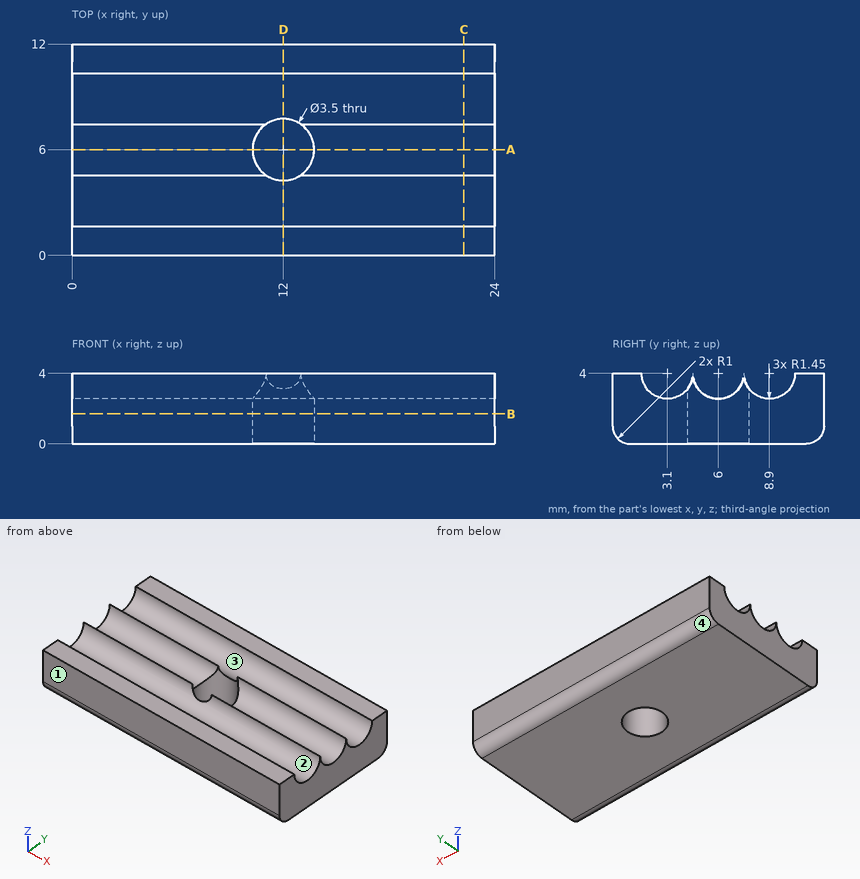
Design review of the part shown in the three views and the two pictorial views. Dimensions are in mm from the part's minimum x, y and z. Round coordinates to 2 decimals unless told otherwise and drop trailing zeros. Write each loop counter-clockwise with the first axis right and the second up, starting at its lowest first coordinate (ties: lowest second). Pieces come first, ordered by that corner, then holes. Notation, with made-up numbers: (53, 2.5) -> (59, 2.5) arc R21 cw to (59, 39.5) -> close; hole circle Ø7 at (87.5, -35.5). An arc over 180 degrees is marked (long way). Use one line per item in the form item = value.
1) Clearance check with a flat-ended pin moving along its axis: pin 1 (2 mm diameter, centred on x = 6, y = 6, fed in from +Z). State where the tip first meets the part, or that it passes through.
Found:
pin_1 = 2.95
2) To check wall thickness, follow L1, parallel to X at y = 6, z = 1.5; L2, parallel to Y at x = 12, z = 2.3; L3, parallel to Y at x = 10.75, z = 2.7. State the ranges of each line that lie inside material, in increasing order. Write a range as from..to.
Found:
L1 = 0..10.25, 13.75..24
L2 = 0..4.25, 7.75..12
L3 = 0..2.46, 3.74..4.78, 7.22..8.26, 9.54..12
3) Take a section at C-C, the plane x = 22.25. Write out the cut boundary in (y, z), and give its area (3 significant figures).
Found:
outline = (0, 1) arc R1 ccw to (1, 0) -> (11, 0) arc R1 ccw to (12, 1) -> (12, 4) -> (10.35, 4) arc R1.45 cw to (7.45, 4) arc R1.45 cw to (4.55, 4) arc R1.45 cw to (1.65, 4) -> (0, 4) -> close
area = 37.7 mm2
4) Take a section at B-B, the plane z = 1.7. Write out the cut boundary in (x, y).
Found:
outline = (0, 0) -> (24, 0) -> (24, 12) -> (0, 12) -> close; hole circle Ø3.5 at (12, 6)
5) Take a section at A-A, the plane y = 6. Write out the cut boundary in (x, z), and give its area (3 significant figures).
Found:
outline = (0, 0) -> (10.25, 0) -> (10.25, 2.55) -> (0, 2.55) -> close; (13.75, 0) -> (24, 0) -> (24, 2.55) -> (13.75, 2.55) -> close
area = 52.3 mm2
6) Take a section at D-D, the plane x = 12. Write out the cut boundary in (y, z).
Found:
outline = (0, 1) arc R1 ccw to (1, 0) -> (4.25, 0) -> (4.25, 3.12) arc R1.45 cw to (1.65, 4) -> (0, 4) -> close; (7.75, 0) -> (11, 0) arc R1 ccw to (12, 1) -> (12, 4) -> (10.35, 4) arc R1.45 cw to (7.75, 3.12) -> close
7) Mouldability with a two-part tool opening along Y and no side actions: class the marked faces 1, 2, 3 and 4 as +Y half, -Y half, draft (parallel to the pull), parting line (faces both ways), or undercut.
Found:
face_1 = -Y half
face_2 = undercut
face_3 = undercut
face_4 = +Y half
